Input: part model. Units: mm. Frame: model coordinates. Face numbers are marked on the shaded views. A direction names the side the tool comes from. Round coordinates to 2 decimals unless told otherwise and drop trailing zeros. Order: outer loops, then holes, each group sorted by start corner. A loop starts at its lowest first (then second) coordinate and runs counter-clockwise, first axis right, second up. Notation, with made-up numbers: (-9.5, -21) -> (35.5, -21) arc R30 ccw to (35.5, 12) -> close; hole circle Ø9 at (-32.75, -4.75). An arc over 180 degrees is marked (long way). Use a Markdown table: item, result.
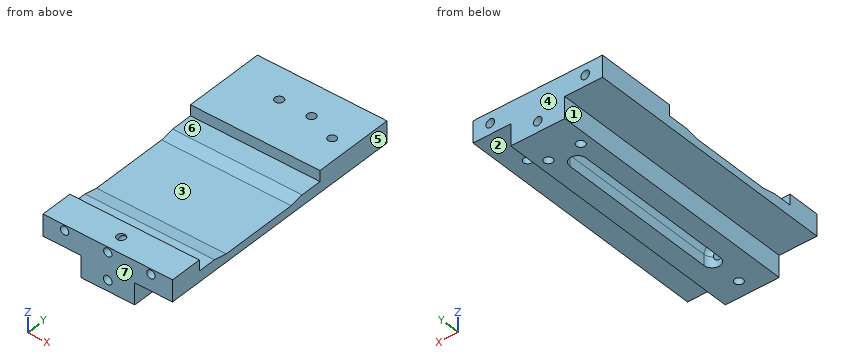
from build123d import *

# Parameters (mm, degrees)
BOSS_EXTRUDE1_DEPTH              = 76.2
CUT_EXTRUDE3_DEPTH               = 47.625
CUT_EXTRUDE4_DEPTH               = 110.433918417
F_10_0_1935_DIAMETER_HOLE1_D     = 4.9149
F_10_0_1935_DIAMETER_HOLE1_DEPTH = 19.05
F_10_0_1935_DIAMETER_HOLE1_TIP   = 1.476584928
F_1_4_20_TAPPED_HOLE1_D          = 5.1054
SKETCH19_R                       = 2.499999953
CUT_EXTRUDE5_DEPTH               = 87.135590889
F_1_4_20_TAPPED_HOLE2_D          = 5.1054
F_1_4_20_TAPPED_HOLE2_DEPTH      = 39.53002
F_1_4_20_TAPPED_HOLE2_TIP        = 1.533816902
F_1_4_20_TAPPED_HOLE3_D          = 5.1054
F_1_4_20_TAPPED_HOLE3_DEPTH      = 42.07002
F_1_4_20_TAPPED_HOLE3_TIP        = 1.533816902


with BuildPart() as part:
    # Sketch1 → Boss-Extrude1 (new, symmetric)
    with BuildSketch(Plane(origin=(0, 0, 0), x_dir=(1, 0, 0), z_dir=(0, 1, 0))):
        Polygon((-15.875, 6.35), (-15.875, 19.05), (15.875, 19.05), (15.875, 6.35), (38.1, 6.35), (38.1, -6.35), (-38.1, -6.35), (-38.1, 6.35), align=None)
    extrude(amount=BOSS_EXTRUDE1_DEPTH, both=True)

    # Sketch5 → Cut-Extrude3 (cut, symmetric)
    with BuildSketch(Plane(origin=(0, 0, 0), x_dir=(1, 0, 0), z_dir=(0, 1, 0))):
        with BuildLine():
            Line((-4.7625, 19.05), (-4.7625, 12.7))
            ThreePointArc((-4.7625, 12.7), (0, 7.9375), (4.7625, 12.7))
            Line((4.7625, 12.7), (4.7625, 19.05))
            Line((4.7625, 19.05), (-4.7625, 19.05))
        make_face()
    extrude(amount=CUT_EXTRUDE3_DEPTH, both=True, mode=Mode.SUBTRACT)

    # Sketch9 → Cut-Revolve1 (revolve, cut)
    with BuildSketch(Plane(origin=(0, 0, 0), x_dir=(0, 0, -1), z_dir=(1, 0, 0))):
        with BuildLine():
            Line((19.05, -52.3875), (12.7, -52.3875))
            ThreePointArc((12.7, -52.3875), (9.332403955, -50.992596045), (7.9375, -47.625))
            Line((7.9375, -47.625), (19.05, -47.625))
            Line((19.05, -47.625), (19.05, -52.3875))
        make_face()
    cut_revolve1 = revolve(axis=Axis((0, -47.625, -7.9375), (0, 0, -1)), mode=Mode.SUBTRACT)

    # Mirror1: Cut-Revolve1 across plane
    add(cut_revolve1.mirror(Plane.ZX), mode=Mode.SUBTRACT)

    # Sketch12 → Cut-Extrude4 (cut, through all)
    with BuildSketch(Plane(origin=(38.1, 0, 0), x_dir=(0, 0, -1), z_dir=(1, 0, 0))):
        Polygon((-6.35, -57.15), (0, -57.15), (0, -46.343697859), (1.5875, -38.1), (1.5875, 8.129025313), (0, 15.875), (0, 28.575), (-6.35, 28.575), align=None)
    extrude(amount=-CUT_EXTRUDE4_DEPTH, mode=Mode.SUBTRACT)

    # #10 (0.1935) Diameter Hole1
    with Locations(Plane(origin=(0, -76.2, 0), x_dir=(-1, 0, 0), z_dir=(0, -1, 0))):
        with Locations((25.4, -3.175), (-25.4, -3.175), (0, -3.175)):
            Hole(F_10_0_1935_DIAMETER_HOLE1_D / 2, depth=F_10_0_1935_DIAMETER_HOLE1_DEPTH)
            with Locations((0, 0, -(F_10_0_1935_DIAMETER_HOLE1_DEPTH + F_10_0_1935_DIAMETER_HOLE1_TIP / 2))):  # 118° drill point
                Cone(0, F_10_0_1935_DIAMETER_HOLE1_D / 2, F_10_0_1935_DIAMETER_HOLE1_TIP, mode=Mode.SUBTRACT)

    # 1/4-20 Tapped Hole1 (through all)
    with Locations(Plane(origin=(0, 76.2, 0), x_dir=(1, 0, 0), z_dir=(0, 1, 0))):
        with Locations((0, 12.7)):
            Hole(F_1_4_20_TAPPED_HOLE1_D / 2)

    # Sketch19 → Cut-Extrude5 (cut, through all)
    with BuildSketch(Plane(origin=(0, 0, -6.35), x_dir=(-1, 0, 0), z_dir=(0, 0, -1))):
        with Locations((-27.209019229, 50.43691079)):
            Circle(SKETCH19_R)
    extrude(amount=-CUT_EXTRUDE5_DEPTH, mode=Mode.SUBTRACT)

    # 1/4-20 Tapped Hole2
    with Locations(Plane(origin=(0, 76.2, 0), x_dir=(1, 0, 0), z_dir=(0, 1, 0))):
        with Locations((27.94, 0), (-27.94, 0)):
            Hole(F_1_4_20_TAPPED_HOLE2_D / 2, depth=F_1_4_20_TAPPED_HOLE2_DEPTH)
            with Locations((0, 0, -(F_1_4_20_TAPPED_HOLE2_DEPTH + F_1_4_20_TAPPED_HOLE2_TIP / 2))):  # 118° drill point
                Cone(0, F_1_4_20_TAPPED_HOLE2_D / 2, F_1_4_20_TAPPED_HOLE2_TIP, mode=Mode.SUBTRACT)

    # 1/4-20 Tapped Hole3
    with Locations(Plane(origin=(0, 0, -19.05), x_dir=(-1, 0, 0), z_dir=(0, 0, -1))):
        with Locations((0, -66.675), (9.525, 57.15), (-9.525, 57.15)):
            Hole(F_1_4_20_TAPPED_HOLE3_D / 2, depth=F_1_4_20_TAPPED_HOLE3_DEPTH)
            with Locations((0, 0, -(F_1_4_20_TAPPED_HOLE3_DEPTH + F_1_4_20_TAPPED_HOLE3_TIP / 2))):  # 118° drill point
                Cone(0, F_1_4_20_TAPPED_HOLE3_D / 2, F_1_4_20_TAPPED_HOLE3_TIP, mode=Mode.SUBTRACT)


solid = part.part
1) Cut plane A-A on y = 57.15. Return loops of the section in (x, z) (3 decimals), and give its area (3 significant figures).
Answer key:
| item | result |
|---|---|
| outline | (-38.1, -6.35) -> (-15.875, -6.35) -> (-15.875, -19.05) -> (-12.078, -19.05) -> (-12.078, 6.35) -> (-38.1, 6.35) -> close; (-6.972, -19.05) -> (6.972, -19.05) -> (6.972, 6.35) -> (-6.972, 6.35) -> close; (12.078, -19.05) -> (15.875, -19.05) -> (15.875, -6.35) -> (38.1, -6.35) -> (38.1, 6.35) -> (12.078, 6.35) -> close; hole circle Ø5.105 at (-27.94, 0); hole circle Ø5.105 at (0, -12.7); hole circle Ø5.105 at (27.94, 0) |
| area | 1,050 mm^2 |
2) Ray query, probe 1 along Z at (x, y) = (0, -69.5); probe 2 along Z at (x, y) = (-27.94, 65.5); probe 3 along Y at (x, z) = (19, 3.75) (3 decimals). Return the intervals inside material, ascending.
Answer key:
| item | result |
|---|---|
| probe 1 | z = -19.05 to -15.25, -10.15 to 0.72, 5.63 to 6.35 |
| probe 2 | z = -6.35 to -2.55, 2.55 to 6.35 |
| probe 3 | y = -76.2 to -57.15, 28.575 to 76.2 |
3) Draft query along Y for the marked faces 4, 5, 6 and 7. Return one class per face: released by +Y, released by -Y, zero draft, split by the parting line, or undercut.
Answer key:
| item | result |
|---|---|
| face 4 | released by +Y |
| face 5 | zero draft |
| face 6 | undercut |
| face 7 | released by -Y |
4) Cut plane D-D on x = 0. State how many separate pieces and enclosed holes the cut face has, and give its area (3 significant figures).
Answer key:
| item | result |
|---|---|
| separate pieces | 7 |
| enclosed holes | 0 |
| area | 1,670 mm^2 |
5) Set-up query: the marked faces 1, 2 and 3. Return all of +Z, -Z, +X, -X, +Y, -Y with unobstructed straight access to the full face (end or side cutting, diameter ignored); none if empty.
Answer key:
| item | result |
|---|---|
| face 1 | -Z, -X, +Y, -Y |
| face 2 | -Z, +X, +Y, -Y |
| face 3 | +Z, +X, -X |
6) Contact query for flat-ended pins moving along their axis: P1, Ø3, axis at x = 9.525, y = 57.15, coming from the -Z side; P2, Ø7, axis at y = -13, z = -15, coming from the +X side (3 decimals); P3, Ø5, axis at y = -13, z = -11.5, coming from the -X side (3 decimals); P4, Ø6.5, axis at x = 27.21, y = 50.44, coming from the -Z side. Output: stop coordinate, or through.
Answer key:
| item | result |
|---|---|
| P1 | passes through |
| P2 | stops at x = 15.875 |
| P3 | stops at x = -15.875 |
| P4 | stops at z = -6.35 |
